Input: part model. Units: mm. Frame: model coordinates. A direction names the side the tool comes from. Round coordinates to 2 decimals unless told otherwise and drop trailing zeros. Loops run counter-clockwise (first coordinate to the right, second up) from the corner with the lowest first, then second, coordinate; pieces in that order, holes last. Notation, with made-up numbers: (80.25, 83.5) - (95.25, 83.5) arc R14 cw to (95.25, 107.5) - close; hole circle Ø4 at (-15.75, 51.25). An arc over 180 degrees is marked (long way). Write each question's results on one line, items separated by ' | '.
from build123d import *

# Parameters (mm, degrees)
F0_W     = 100
F0_H     = 100
F1_DEPTH = 100
F6_R     = 5
F7_DEPTH = 50.001


# Not quite as in the source:
# - a feature of the source that left no trace in its solid (it failed there, or was rolled back) is left out


with BuildPart() as f1:
    # F0 (on Front) → F1 (new body)
    with BuildSketch(Plane.XZ):
        Rectangle(F0_W, F0_H)
    extrude(amount=F1_DEPTH)

    # F6 (on Right) → F7 (cut, through all)
    with BuildSketch(Plane.YZ):
        with Locations((-17.9369883015, 0)):
            Circle(F6_R)
    extrude(amount=-F7_DEPTH, mode=Mode.SUBTRACT)


solid = f1.part
1. Set-up query: faces 1 (the flat face through (-1, 0, 1)), 2 (the cylindrical face through (-24.65, -13.168, 1.502)). Return all of +Z, -Z, +X, -X, +Y, -Y with unobstructed straight access to the full face (end or side cutting, diameter ignored); none if empty.
Answer:
face 1: +Z, -Z, +X, -X, +Y | face 2: -X
2. Section query B-B, the plane y = -17.5. Output: boundary loops of the cut face in (x, z), plus the area to 3 significant figures.
Answer:
outline: (-50, -50) - (50, -50) - (50, 50) - (-50, 50) - (-50, 4.98) - (0, 4.98) - (0, -4.98) - (-50, -4.98) - close | area: 9,500 mm^2
3. Mould query, pull axis Z, two halves, no side actions, for faces 3 (the flat face through (-1, -49, -50)), 4 (the flat face through (50, -49, -1)), 5 (the flat face through (0, -18, 0)). Classes: pulls with the +Z half, pulls with the -Z half, needs draft (parallel to the pull), parting line crosses it, or undercut.
Answer:
face 3: pulls with the -Z half | face 4: needs draft | face 5: undercut
4. Section query A-A, the plane z = 0. Output: boundary loops of the cut face in (x, y), plus the area to 3 significant figures.
Answer:
outline: (-50, -100) - (50, -100) - (50, 0) - (-50, 0) - (-50, -12.94) - (0, -12.94) - (0, -22.94) - (-50, -22.94) - close | area: 9,500 mm^2
5. Line query: line 1 (X direction, y = -15, z = 4); line 2 (Z direction, x = -3, y = -13.5). Output: solid intervals per line, ascending. Write a range as [from, to].
Answer:
line 1: [0, 50] | line 2: [-50, -2.31], [2.31, 50]
